For this review, take the finished solid that the model builds, in its own axes (mm). A direction names the side the tool comes from. Round coordinates to 2 decimals unless told otherwise and drop trailing zeros. Write each loop counter-clockwise with the first axis right and the second up, starting at its lowest first coordinate (ties: lowest second). Pieces come first, ordered by that corner, then holes. Notation, with made-up numbers: M 60,-21 L 90,-21 A7 ccw 90,-12 Z; hole C 59.5,10 d1. An arc over 180 degrees is marked long. Use one line per item in the form item = value. Start each with the question number.
Item 1: Add section D-D (z = -35). State the section outline as (x, y) points (3 decimals), and give its area (3 significant figures).
Item 2: For faces 5 (the flat face through (1.35, 9, 37)), 6 (the flat face through (-6.35, 9, -17)), 7 (the flat face through (-2, 12.7, 17)), 8 (the cylindrical face through (-1.201, 1.983, -23.815)), list the 3-axis set-ups (+Z, -Z, +X, -X, +Y, -Y) from which the entire face can be reached by the end or side of a thin tool; tool diameter is ignored.
Item 3: Draft analysis for pull direction Z (two halves, no side actions). For faces 1 (the flat face through (-8.815, 6.261, 10.465)), 2 (the cylindrical face through (3.874, 2.971, 23.685)), 3 (the flat face through (-2, 6, 42)), 4 (the cylindrical face through (2.4, 2, -31.8)), state which applies: released by +Z, released by -Z, zero draft, split by the parting line, or undercut.
Item 4: For line 1 (Z direction, x = 0, y = 1.9); line 2 (Y direction, x = -7, z = 20); line 3 (X direction, y = 13, z = -20), list the stretches that pass through material, from the lowest coordinate up. Write a range as [from, to].
Item 5: For P1, Ø3, axis at x = -5.5, y = 15, coming from the +Z side; P2, Ø6.5, axis at x = 0, z = -35, coming from the -Y side; P3, Ø9, axis at y = 6.35, z = 20, coming from the +X side, all flat-tipped, find the tip position at first contact; note any pin that passes through.
Item 6: Add section A-A (z = 20). State the section outline as (x, y) points (3 decimals), and give its area (3 significant figures).
Item 7: Add section B-B (x = 0). Count the separate pieces of the cut face and the enclosed holes in it, and give its area (3 significant figures).
from build123d import *

# Parameters (mm, degrees)
SKETCH2_W                     = 12.7
SKETCH2_H                     = 84
BOSS_EXTRUDE1_DEPTH           = 12.7
SKETCH5_W                     = 12.7
SKETCH5_H                     = 29
BOSS_EXTRUDE2_DEPTH           = 5
CBORE_FOR_M4_SHCS1_AT_2_COUNT = 2
CBORE_FOR_M4_SHCS1_AT_2_PITCH = 15
SKETCH8_W                     = 29
SKETCH8_H                     = 12.7
BOSS_EXTRUDE3_DEPTH           = 5
CBORE_FOR_M5_SHCS2_AT_2_COUNT = 2
CBORE_FOR_M5_SHCS2_AT_2_PITCH = 15
CHAMFER1_SIZE                 = 5


with BuildPart() as part:
    # Sketch2 → Boss-Extrude1 (new body)
    with BuildSketch(Plane(origin=(0, 0, 0), x_dir=(1, 0, 0), z_dir=(0, 1, 0))):
        Rectangle(SKETCH2_W, SKETCH2_H)
    extrude(amount=BOSS_EXTRUDE1_DEPTH)

    # Sketch5 → Boss-Extrude2 (add)
    with BuildSketch(Plane(origin=(0, 12.7, 0), x_dir=(1, 0, 0), z_dir=(0, 1, 0))):
        with Locations((0, 27.5)):
            Rectangle(SKETCH5_W, SKETCH5_H)
    extrude(amount=BOSS_EXTRUDE2_DEPTH)

    # Sketch4 → CBORE for M4 SHCS1 (revolve, cut)
    with BuildSketch(Plane(origin=(0, 0, -35), x_dir=(0, 0, -1), z_dir=(1, 0, 0))):
        Polygon((0, 0), (0, 17.7), (2.4, 17.7), (2.4, 4), (4, 4), (4, 0.020977491), (4.025, 0), align=None)
    cbore_for_m4_shcs1 = revolve(axis=Axis((0, -6.35, -35), (0, 1, 0)), mode=Mode.SUBTRACT)

    # CBORE for M4 SHCS1 at 2: CBORE for M4 SHCS1 ×2
    with Locations(*[(0, 0, i * CBORE_FOR_M4_SHCS1_AT_2_PITCH) for i in range(1, CBORE_FOR_M4_SHCS1_AT_2_COUNT)]):
        add(cbore_for_m4_shcs1, mode=Mode.SUBTRACT)

    # Sketch8 → Boss-Extrude3 (add)
    with BuildSketch(Plane.ZY.offset(6.35)):
        with Locations((27.5, 6.35)):
            Rectangle(SKETCH8_W, SKETCH8_H)
    extrude(amount=BOSS_EXTRUDE3_DEPTH)

    # Sketch7 → CBORE for M5 SHCS2 (revolve, cut)
    with BuildSketch(Plane(origin=(6.35, 6.35, 35), x_dir=(0, 0, -1), z_dir=(0, 1, 0))):
        Polygon((0, 0), (0, 17.7), (2.9, 17.7), (2.9, 5), (5, 5), (5, 0.020977491), (5.025, 0), align=None)
    cbore_for_m5_shcs2 = revolve(axis=Axis((12.7, 6.35, 35), (-1, 0, 0)), mode=Mode.SUBTRACT)

    # CBORE for M5 SHCS2 at 2: CBORE for M5 SHCS2 ×2
    with Locations(*[(0, 0, -i * CBORE_FOR_M5_SHCS2_AT_2_PITCH) for i in range(1, CBORE_FOR_M5_SHCS2_AT_2_COUNT)]):
        add(cbore_for_m5_shcs2, mode=Mode.SUBTRACT)

    # Chamfer1
    chamfer1_edges = [part.edges().sort_by_distance(p)[0] for p in [
        (0, 12.7, -13),
        (-6.35, 6.35, 13),
    ]]
    chamfer(chamfer1_edges, length=CHAMFER1_SIZE - 0.0001)  # a hair under: the kernel refuses the full size


solid = part.part
Calculated:
q1.outline = M -6.35,0 L -4.025,0 L -4,0.021 L -4,4 L -2.4,4 L -2.4,17.7 L -6.35,17.7 Z; M 2.4,4 L 4,4 L 4,0.021 L 4.025,0 L 6.35,0 L 6.35,17.7 L 2.4,17.7 Z
q1.area = 127 mm^2
q2.face_5 = +X
q2.face_6 = -Z, -X, +Y, -Y
q2.face_7 = +Z, +X, -X, +Y
q2.face_8 = -Y
q3.face_1 = released by -Z
q3.face_2 = undercut
q3.face_3 = released by +Z
q3.face_4 = undercut
q4.line_1 = [-42, -39], [-31, -24], [-16, 42]
q4.line_2 = [0, 3.45], [9.25, 12.7]
q4.line_3 = [-6.35, -2.4], [2.4, 6.35]
q5.P1 = -8.8
q5.P2 = 4
q5.P3 = 1.35
q6.outline = M -11.35,0 L 6.35,0 L 6.35,1.325 L 6.329,1.35 L 1.35,1.35 L 1.35,3.45 L -11.35,3.45 Z; M -11.35,9.25 L 1.35,9.25 L 1.35,11.35 L 6.329,11.35 L 6.35,11.375 L 6.35,12.7 L -11.35,12.7 Z
q6.area = 101 mm^2
q7.separate_pieces = 3
q7.enclosed_holes = 2
q7.area = 976 mm^2
